The model under review builds one solid part; all positions refer to its coordinate system, in mm. Face numbers are marked on the shaded views. Round coordinates to 2 decimals unless told otherwise and drop trailing zeros. Order: outer loops, then holes, each group sorted by start corner. A loop starts at its lowest first (then second) coordinate and runs counter-clockwise, first axis right, second up. Notation, with made-up numbers: M 89.5,10 L 131.5,10 A36 ccw 131.5,45 Z; hole C -38,-24.75 d5. An arc over 180 degrees is marked long. Answer as a JSON object with one key per item and string values. Group by question number.
1) Consider section C-C, the plane z = 2. Write out the cut boundary in (x, y), then the cut area to 3 significant figures.
2) Consider section B-B, the plane x = 15. Write out the cut boundary in (y, z), then the cut area to 3 significant figures.
3) Insertion check: pin 1 Ø1.6 at (y, z) = (-7.5, 11.5) entering from +X (3 decimals); pin 2 Ø1.6 at (y, z) = (-15.5, 11) entering from -X; pin 3 Ø2 at (y, z) = (-8, 10) entering from -X. Each pin has a flat end and moves straight along its axis. Give the tip position at first contact, or say it passes through.
4) To check wall thickness, follow line 1 (Z direction, x = 21, y = -16); line 2 (X direction, y = -3.5, z = 11.5); line 3 (X direction, y = -22.75, z = 7). State the ranges of each line that lie inside material, in increasing order.
5) The part is to be moulded in two halves that separate along Z. For the marked faces 1, 2 and 3, say which applies: +Z half, -Z half, draft (parallel to the pull), parting line (faces both ways), or undercut.
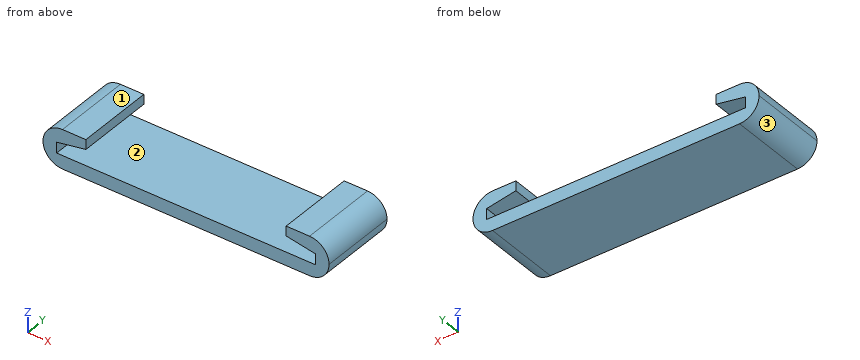
```python
from build123d import *

# Parameters (mm, degrees)
F1_DEPTH = 25.4
F2_R     = 6.34999


# Not quite as in the source:
# - a fillet or chamfer is up to 0.001 mm smaller than in the source, because OpenCascade refuses the exact size


with BuildPart() as f1:
    # F0 (on Front) → F1 (new body)
    with BuildSketch(Plane.XZ):
        Polygon((-46.609, 0), (0, 0), (0, 4.3402855088), (-42.164, 4.3402855088), (-42.164, 7.8454855088), (-32.639, 9.525), (-32.639, 12.7), (-46.609, 12.7), align=None)
    extrude(amount=F1_DEPTH)

    # F2 (radius 6.35 in the source; OpenCascade refuses exactly that, so slightly less here)
    f2_edges = [f1.edges().sort_by_distance(p)[0] for p in [
        (-46.609, -12.7, 12.7),
        (-46.609, -12.7, 0),
    ]]
    fillet(f2_edges, radius=F2_R)

    # F3: F1 across face


with BuildPart() as f1_1:
    add(f1.part)
    add(f1.part.mirror(Plane(origin=(0, -12.7, 2.1701427544), x_dir=(0, 1, 0), z_dir=(1, 0, 0))))


solid = f1_1.part
```
Results list:
{
 "1": {"outline": "M -44.89,-25.4 L 44.89,-25.4 L 44.89,0 L -44.89,0 Z", "area": "2,280 mm^2"},
 "2": {"outline": "M -25.4,0 L 0,0 L 0,4.34 L -25.4,4.34 Z", "area": "110 mm^2"},
 "3": {"pin 1": "x = 44.885", "pin 2": "x = -45.31", "pin 3": "x = -46.03"},
 "4": {"line 1": "0 to 4.34", "line 2": "-43.97 to -32.64, 32.64 to 43.97", "line 3": "-46.58 to -42.16, 42.16 to 46.58"},
 "5": {"face 1": "+Z half", "face 2": "undercut", "face 3": "-Z half"}
}
